The model under review builds one solid part; all positions refer to its coordinate system, in mm. A direction names the side the tool comes from. Coordinates: 2 decimals unless noted, no trailing zeros. Loops run counter-clockwise (first coordinate to the right, second up) from the corner with the lowest first, then second, coordinate; pieces in that order, holes last. Notation, with made-up numbers: (49.5, 88.25) - (77.5, 88.25) arc R18 ccw to (77.5, 122.25) - close; hole circle Ø1 at (16, 37.5). An arc over 180 degrees is marked (long way). Answer in a Markdown table with one row per item. Add a question column.
(1) We need section B-B on z = 32.5. Write out the cut boundary in (x, y).
(2) We need section A-A on z = 144. Write out the cut boundary in (x, y).
(3) We need section D-D on y = 10.5. Write out the cut boundary in (x, z), plus the area to 3 significant figures.
(4) Machinability: for faces 1 (the cylindrical face through (20.29, 19.74, 12.34)), 2 (the flat face through (-29, 35.352, 74)), 3 (the cylindrical face through (-12.69, 39.3, 4.45)), which of the approach directions +Z, -Z, +X, -X, +Y, -Y give a long, thin tool a straight path to every point of the face, cutting with its end or side? Answer none if there is none.
(5) For P1, Ø21, axis at x = -27.5, z = 104, coming from the -Y side; P2, Ø1.5, axis at y = 7.5, z = 15, coming from the +X side, all flat-tipped, find the tip position at first contact; note any pin that passes through.
(6) Mouldability with a two-part tool opening along Z and no side actions: class faces 4 (the flat face through (-12, 37, 150)), 5 (the flat face through (-2.501, 12, 74)), 6 (the cylindrical face through (20.289, 19.965, 137.53)), 7 (the cylindrical face through (20.289, 17.962, 47.974)) as +Z half, -Z half, draft (parallel to the pull), parting line (faces both ways), or undercut.
(7) We need section C-C on x = -37. Write out the cut boundary in (y, z), plus the area to 3 significant figures.
(8) For line 1 along X through (y, z) = (38, 144); line 2 along X through (y, z) = (13, 96); line 3 along Y through (x, z) = (-13.5, 86.5), list the stretches that pass through material, from the lowest coordinate up.
from build123d import *

# Parameters (mm, degrees)
F1_DEPTH = 150
F2_R     = 3
F3_DEPTH = 30
F4_R     = 1.75
F5_DEPTH = 8


with BuildPart() as f1:
    # F0 (on Top) → F1 (new body)
    with BuildSketch(Plane.XY):
        with BuildLine():
            Line((-49.501332, 43.352309), (-49.501332, 35.352309))
            Line((-49.501332, 35.352309), (-7.501332, 35.352309))
            ThreePointArc((-7.501332, 35.352309), (-3.965798, 33.887843), (-2.501332, 30.352309))
            Line((-2.501332, 30.352309), (-2.501332, -6.647691))
            Line((-2.501332, -6.647691), (5.498668, -6.647691))
            Line((5.498668, -6.647691), (5.498668, 43.352309))
            Line((5.498668, 43.352309), (-49.501332, 43.352309))
        make_face()
    extrude(amount=F1_DEPTH)

    # F2 (on face) → F3 (join)
    with BuildSketch(Plane.YZ.offset(5.498668)):
        with Locations((18.352309, 135)):
            Circle(F2_R)
        with Locations((18.352309, 105)):
            Circle(F2_R)
        with Locations((18.352309, 75)):
            Circle(F2_R)
        with Locations((18.352309, 45)):
            Circle(F2_R)
        with Locations((18.352309, 15)):
            Circle(F2_R)
    extrude(amount=F3_DEPTH)

    # F4 (on face) → F5 (cut)
    with BuildSketch(Plane.XZ.offset(-35.352309)):
        with Locations((-43.501332, 6)):
            Circle(F4_R)
        with Locations((-13.501332, 6)):
            Circle(F4_R)
        with Locations((-43.501332, 144)):
            Circle(F4_R)
        with Locations((-13.501332, 144)):
            Circle(F4_R)
    extrude(amount=-F5_DEPTH, mode=Mode.SUBTRACT)


solid = f1.part
Outcome:
| question | item | result |
|---|---|---|
| 1 | outline | (-49.5, 35.35) - (-7.5, 35.35) arc R5 cw to (-2.5, 30.35) - (-2.5, -6.65) - (5.5, -6.65) - (5.5, 43.35) - (-49.5, 43.35) - close |
| 2 | outline | (-49.5, 35.35) - (-45.25, 35.35) - (-45.25, 43.35) - (-49.5, 43.35) - close; (-41.75, 35.35) - (-15.25, 35.35) - (-15.25, 43.35) - (-41.75, 43.35) - close; (-11.75, 35.35) - (-7.5, 35.35) arc R5 cw to (-2.5, 30.35) - (-2.5, -6.65) - (5.5, -6.65) - (5.5, 43.35) - (-11.75, 43.35) - close |
| 3 | outline | (-2.5, 0) - (5.5, 0) - (5.5, 150) - (-2.5, 150) - close |
| 3 | area | 1,200 mm² |
| 4 | face 1 | +X |
| 4 | face 2 | +Z, -Z, -X, -Y |
| 4 | face 3 | +Y, -Y |
| 5 | P1 | y = 35.35 |
| 5 | P2 | x = 5.5 |
| 6 | face 4 | +Z half |
| 6 | face 5 | draft |
| 6 | face 6 | undercut |
| 6 | face 7 | undercut |
| 7 | outline | (35.35, 0) - (43.35, 0) - (43.35, 150) - (35.35, 150) - close |
| 7 | area | 1,200 mm² |
| 8 | line 1 | -49.5 to -45.25, -41.75 to -15.25, -11.75 to 5.5 |
| 8 | line 2 | -2.5 to 5.5 |
| 8 | line 3 | 35.35 to 43.35 |
